Geometry check sheet. Reference: the model listing, model coordinates, mm. A direction names the side the tool comes from. Give positions to 0.01 mm unless a question says otherwise; leave off trailing zeros. Loops run counter-clockwise (first coordinate to the right, second up) from the corner with the lowest first, then second, coordinate; pieces in that order, holes last. Notation, with made-up numbers: (-18.5, 61.25) - (-2.5, 61.25) arc R20 cw to (-2.5, 73.25) - close; hole circle Ø3 at (33, 87). An arc over 180 degrees is marked (long way). Write item = value, one per line. Start each with the question number.
from build123d import *

# Parameters (mm, degrees)
SKETCH11_R          = 1.75
SKETCH8_R           = 1.75
BOSS_EXTRUDE1_DEPTH = 3.5
FILLET1_R           = 2
FILLET2_R           = 2


with BuildPart() as part:
    # Sweep1: sweep along a path in Sketch1
    with BuildLine(Plane(origin=(0, 0, 0), x_dir=(1, 0, 0), z_dir=(0, 1, 0))) as sweep1_path:
        Line((0, 0), (-4.736065928, -1.093406974))
        ThreePointArc((-4.736065928, -1.093406974), (-5.853544334, -1.285424883), (-6.985576472, -1.349706326))
        Line((-6.985576472, -1.349706326), (-210.672794298, -1.349706326))
        ThreePointArc((-210.672794298, -1.349706326), (-212.323270357, -1.212562341), (-213.928475842, -0.804892082))
        Line((-213.928475842, -0.804892082), (-226.582134244, 3.552111915))
        ThreePointArc((-226.582134244, 3.552111915), (-228.446084779, 3.999606846), (-230.361175351, 4.083221506))
        Line((-230.361175351, 4.083221506), (-249.305198661, 3.090407314))
        ThreePointArc((-249.305198661, 3.090407314), (-251.788897094, 2.641281474), (-254.081031741, 1.584592928))
        Line((-254.081031741, 1.584592928), (-268.848792164, -7.643327957))
    # Sketch11 → Sweep1 (sweep)
    with BuildSketch(Plane(origin=(0, 0, 0), x_dir=(0.22495105434386561, 0, 0.9743700647852351), z_dir=(-0.9743700647852351, 0, 0.22495105434386561))):
        Circle(SKETCH11_R)
    sweep(path=sweep1_path.line)

    # Sweep3: sweep along a curve in space
    with BuildLine() as sweep3_path:
        Line((-272.410594168, -3, 9.868988866), (-272.410594168, -8, 9.868988866))
        ThreePointArc((-269.866449879, 0, 8.279231074), (-271.665431558, -0.878679656, 9.403359589), (-272.410594168, -3, 9.868988866))
        Line((-269.866449879, 0, 8.279231074), (-268.848792164, 0, 7.643327957))
    # Sketch8 → Sweep3 (sweep)
    with BuildSketch(Plane(origin=(-196.787061579, 0, 122.966203633), x_dir=(0.5299192642332071, 0, 0.8480480961564246), z_dir=(-0.8480480961564246, 0, 0.5299192642332071))):
        with Locations((-135.986244411, 0)):
            Circle(SKETCH8_R)
    sweep(path=sweep3_path.line)

    # Sketch5 → Boss-Extrude1 (add, symmetric)
    with BuildSketch(Plane(origin=(0, 0, 0), x_dir=(1, 0, 0), z_dir=(0, 1, 0))):
        with BuildLine():
            Line((-0.393664345, 1.705147613), (19.813870271, 14.370895509))
            ThreePointArc((19.813870271, 14.370895509), (20.700469104, 14.828681695), (21.650674926, 15.133205221))
            Line((21.650674926, 15.133205221), (62.574217647, 24.581149504))
            ThreePointArc((62.574217647, 24.581149504), (64.838828602, 24.202183598), (66.172181004, 22.332892472))
            Line((66.172181004, 22.332892472), (69.265258001, 8.935304082))
            ThreePointArc((69.265258001, 8.935304082), (68.886292095, 6.670693126), (67.01700097, 5.337340724))
            Line((67.01700097, 5.337340724), (26.093458249, -4.110603558))
            ThreePointArc((26.093458249, -4.110603558), (25.105924586, -4.253442442), (24.108374578, -4.230646291))
            Line((24.108374578, -4.230646291), (0.393664345, -1.705147613))
            Line((0.393664345, -1.705147613), (-0.393664345, 1.705147613))
        make_face()
    extrude(amount=BOSS_EXTRUDE1_DEPTH, both=True)

    # Fillet1
    # the kernel refuses this fillet: 2 mm, written as the material it takes off along each edge
    with BuildSketch(Plane(origin=(23.000381252, 3.5, -9.286984832), x_dir=(-0.5310851635150788, 0, -0.8473184460957769), z_dir=(-0.8473184460957769, 0, 0.5310851635150788))) as fillet1_piece_1:
        with BuildLine():
            CenterArc((6 - FILLET1_R, FILLET1_R), FILLET1_R, 270, 90)
            Line((6, FILLET1_R), (6, 0))
            Line((6, 0), (6 - FILLET1_R, 0))
        make_face()
    revolve(axis=Axis((23.000381252, 3.5, -9.286984832), (0, -1, 0)), revolution_arc=19.078804313, mode=Mode.SUBTRACT)
    with BuildSketch(Plane(origin=(-4.630256576, 3.5, 0.950278204), x_dir=(0, -1, 0), z_dir=(0.8473184460957748, 0, -0.5310851635150823))) as fillet1_piece_2_section:
        with BuildLine():
            CenterArc((FILLET1_R, -FILLET1_R), FILLET1_R, 90, 90)
            Line((0, -FILLET1_R), (0, 0))
            Line((0, 0), (FILLET1_R, 0))
        make_face()
    fillet1_piece_2 = extrude(amount=28.848807622, mode=Mode.PRIVATE)
    fillet1_piece_2 = split(fillet1_piece_2, bisect_by=Plane(origin=(-1.099290547, 3.044511154, -4.761550481), z_dir=(0.9743700647852351, 0, -0.22495105434386561)), keep=Keep.TOP, mode=Mode.PRIVATE)
    add(fillet1_piece_2, mode=Mode.SUBTRACT)
    with BuildSketch(Plane(origin=(1.518419617, 3.5, 6.576997937), x_dir=(0, -1, 0), z_dir=(-0.22495105434386561, 0, -0.9743700647852351))) as fillet1_piece_3_section:
        with BuildLine():
            CenterArc((FILLET1_R, -FILLET1_R), FILLET1_R, 90, 90)
            Line((0, -FILLET1_R), (0, 0))
            Line((0, 0), (FILLET1_R, 0))
        make_face()
    fillet1_piece_3 = extrude(amount=13.5, mode=Mode.PRIVATE)
    fillet1_piece_3 = fillet1_piece_3 - Plane(origin=(0.460325238, 0, -0.106274455), x_dir=(0.22495105434386553, 0, 0.9743700647852351), z_dir=(-0.9743700647852351, 0, 0.22495105434386553)) * Cylinder(1.75, 36, mode=Mode.PRIVATE)
    add(fillet1_piece_3, mode=Mode.SUBTRACT)
    with BuildSketch(Plane(origin=(24.108374578, 3.5, 4.230646291), x_dir=(0, -1, 0), z_dir=(-0.9943771868431155, 0, -0.10589622413463053))) as fillet1_piece_4_section:
        with BuildLine():
            CenterArc((FILLET1_R, -FILLET1_R), FILLET1_R, 90, 90)
            Line((0, -FILLET1_R), (0, 0))
            Line((0, 0), (FILLET1_R, 0))
        make_face()
    fillet1_piece_4 = extrude(amount=28.848807622, mode=Mode.PRIVATE)
    fillet1_piece_4 = split(fillet1_piece_4, bisect_by=Plane(origin=(1.099289941, 3.044511564, 4.761547859), z_dir=(0.9743700647852351, 0, -0.22495105434386561)), keep=Keep.TOP, mode=Mode.PRIVATE)
    add(fillet1_piece_4, mode=Mode.SUBTRACT)
    with BuildSketch(Plane(origin=(24.743751923, 3.5, -1.73561683), x_dir=(0.22495105434386634, 0, 0.9743700647852349), z_dir=(0.9743700647852349, 0, -0.22495105434386634))) as fillet1_piece_5:
        with BuildLine():
            CenterArc((6 - FILLET1_R, FILLET1_R), FILLET1_R, 270, 90)
            Line((6, FILLET1_R), (6, 0))
            Line((6, 0), (6 - FILLET1_R, 0))
        make_face()
    revolve(axis=Axis((24.743751923, 3.5, -1.73561683), (0, -1, 0)), revolution_arc=19.078804313, mode=Mode.SUBTRACT)
    with BuildSketch(Plane(origin=(67.01700097, 3.5, -5.337340724), x_dir=(-0.22495105434386584, 0, -0.9743700647852351), z_dir=(-0.9743700647852351, 0, 0.22495105434386584)), Plane(origin=(21.650674926, 3.5, -15.133205221), x_dir=(0.22495105434386575, 0, 0.974370064785235), z_dir=(0.9743700647852351, 0, -0.22495105434386578))) as fillet1_piece_6:
        with BuildLine():
            CenterArc((FILLET1_R, FILLET1_R), FILLET1_R, 180, 90)
            Line((0, FILLET1_R), (0, 0))
            Line((0, 0), (FILLET1_R, 0))
        make_face()
    extrude(amount=42, mode=Mode.SUBTRACT)
    with BuildSketch(Plane(origin=(66.342147807, 3.5, -8.260450918), x_dir=(0.9743700647852359, 0, -0.22495105434386237), z_dir=(-0.22495105434386237, 0, -0.9743700647852359))) as fillet1_piece_7:
        with BuildLine():
            CenterArc((3 - FILLET1_R, FILLET1_R), FILLET1_R, 270, 90)
            Line((3, FILLET1_R), (3, 0))
            Line((3, 0), (3 - FILLET1_R, 0))
        make_face()
    revolve(axis=Axis((66.342147807, 3.5, -8.260450918), (0, -1, 0)), revolution_arc=90, mode=Mode.SUBTRACT)
    with BuildSketch(Plane(origin=(66.172181004, 3.5, -22.332892472), x_dir=(-0.9743700647852351, 0, 0.22495105434386561), z_dir=(0.2249510543438656, 0, 0.9743700647852351))) as fillet1_piece_8:
        with BuildLine():
            CenterArc((FILLET1_R, FILLET1_R), FILLET1_R, 180, 90)
            Line((0, FILLET1_R), (0, 0))
            Line((0, 0), (FILLET1_R, 0))
        make_face()
    extrude(amount=13.75, mode=Mode.SUBTRACT)
    with BuildSketch(Plane(origin=(63.24907081, 3.5, -21.658039309), x_dir=(-0.22495105434387033, 0, -0.974370064785234), z_dir=(-0.974370064785234, 0, 0.22495105434387033))) as fillet1_piece_9:
        with BuildLine():
            CenterArc((3 - FILLET1_R, FILLET1_R), FILLET1_R, 270, 90)
            Line((3, FILLET1_R), (3, 0))
            Line((3, 0), (3 - FILLET1_R, 0))
        make_face()
    revolve(axis=Axis((63.24907081, 3.5, -21.658039309), (0, -1, 0)), revolution_arc=90, mode=Mode.SUBTRACT)

    # Fillet2
    # the kernel refuses this fillet: 2 mm, written as the material it takes off along each edge
    with BuildSketch(Plane(origin=(23.000381252, -3.5, -9.286984832), x_dir=(-0.5310851635150788, 0, -0.8473184460957769), z_dir=(-0.8473184460957769, 0, 0.5310851635150788))) as fillet2_piece_1:
        with BuildLine():
            CenterArc((6 - FILLET2_R, -FILLET2_R), FILLET2_R, 0, 90)
            Line((6, -FILLET2_R), (6, 0))
            Line((6, 0), (6 - FILLET2_R, 0))
        make_face()
    revolve(axis=Axis((23.000381252, -3.5, -9.286984832), (0, -1, 0)), revolution_arc=19.078804313, mode=Mode.SUBTRACT)
    with BuildSketch(Plane(origin=(-4.630256576, -3.5, 0.950278204), x_dir=(0, 1, 0), z_dir=(0.8473184460957748, 0, -0.5310851635150823))) as fillet2_piece_2_section:
        with BuildLine():
            CenterArc((FILLET2_R, FILLET2_R), FILLET2_R, 180, 90)
            Line((0, FILLET2_R), (0, 0))
            Line((0, 0), (FILLET2_R, 0))
        make_face()
    fillet2_piece_2 = extrude(amount=28.848807622, mode=Mode.PRIVATE)
    fillet2_piece_2 = split(fillet2_piece_2, bisect_by=Plane(origin=(-1.099290547, -3.044511154, -4.761550481), z_dir=(0.9743700647852351, 0, -0.22495105434386561)), keep=Keep.TOP, mode=Mode.PRIVATE)
    add(fillet2_piece_2, mode=Mode.SUBTRACT)
    with BuildSketch(Plane(origin=(1.518419617, -3.5, 6.576997937), x_dir=(0, 1, 0), z_dir=(-0.22495105434386561, 0, -0.9743700647852351))) as fillet2_piece_3_section:
        with BuildLine():
            CenterArc((FILLET2_R, FILLET2_R), FILLET2_R, 180, 90)
            Line((0, FILLET2_R), (0, 0))
            Line((0, 0), (FILLET2_R, 0))
        make_face()
    fillet2_piece_3 = extrude(amount=13.5, mode=Mode.PRIVATE)
    fillet2_piece_3 = fillet2_piece_3 - Plane(origin=(0.460325238, 0, -0.106274455), x_dir=(0.22495105434386553, 0, 0.9743700647852351), z_dir=(-0.9743700647852351, 0, 0.22495105434386553)) * Cylinder(1.75, 36, mode=Mode.PRIVATE)
    add(fillet2_piece_3, mode=Mode.SUBTRACT)
    with BuildSketch(Plane(origin=(24.108374578, -3.5, 4.230646291), x_dir=(0, 1, 0), z_dir=(-0.9943771868431155, 0, -0.10589622413463053))) as fillet2_piece_4_section:
        with BuildLine():
            CenterArc((FILLET2_R, FILLET2_R), FILLET2_R, 180, 90)
            Line((0, FILLET2_R), (0, 0))
            Line((0, 0), (FILLET2_R, 0))
        make_face()
    fillet2_piece_4 = extrude(amount=28.848807622, mode=Mode.PRIVATE)
    fillet2_piece_4 = split(fillet2_piece_4, bisect_by=Plane(origin=(1.099289941, -3.044511564, 4.761547859), z_dir=(0.9743700647852351, 0, -0.22495105434386561)), keep=Keep.TOP, mode=Mode.PRIVATE)
    add(fillet2_piece_4, mode=Mode.SUBTRACT)
    with BuildSketch(Plane(origin=(24.743751923, -3.5, -1.73561683), x_dir=(0.22495105434386634, 0, 0.9743700647852349), z_dir=(0.9743700647852349, 0, -0.22495105434386634))) as fillet2_piece_5:
        with BuildLine():
            CenterArc((6 - FILLET2_R, -FILLET2_R), FILLET2_R, 0, 90)
            Line((6, -FILLET2_R), (6, 0))
            Line((6, 0), (6 - FILLET2_R, 0))
        make_face()
    revolve(axis=Axis((24.743751923, -3.5, -1.73561683), (0, -1, 0)), revolution_arc=19.078804313, mode=Mode.SUBTRACT)
    with BuildSketch(Plane(origin=(67.01700097, -3.5, -5.337340724), x_dir=(-0.22495105434386584, 0, -0.9743700647852351), z_dir=(-0.9743700647852351, 0, 0.22495105434386584)), Plane(origin=(21.650674926, -3.5, -15.133205221), x_dir=(0.22495105434386575, 0, 0.974370064785235), z_dir=(0.9743700647852351, 0, -0.22495105434386578))) as fillet2_piece_6:
        with BuildLine():
            CenterArc((FILLET2_R, -FILLET2_R), FILLET2_R, 90, 90)
            Line((0, -FILLET2_R), (0, 0))
            Line((0, 0), (FILLET2_R, 0))
        make_face()
    extrude(amount=42, mode=Mode.SUBTRACT)
    with BuildSketch(Plane(origin=(66.342147807, -3.5, -8.260450918), x_dir=(0.9743700647852359, 0, -0.22495105434386237), z_dir=(-0.22495105434386237, 0, -0.9743700647852359))) as fillet2_piece_7:
        with BuildLine():
            CenterArc((3 - FILLET2_R, -FILLET2_R), FILLET2_R, 0, 90)
            Line((3, -FILLET2_R), (3, 0))
            Line((3, 0), (3 - FILLET2_R, 0))
        make_face()
    revolve(axis=Axis((66.342147807, -3.5, -8.260450918), (0, -1, 0)), revolution_arc=90, mode=Mode.SUBTRACT)
    with BuildSketch(Plane(origin=(66.172181004, -3.5, -22.332892472), x_dir=(-0.9743700647852351, 0, 0.22495105434386561), z_dir=(0.2249510543438656, 0, 0.9743700647852351))) as fillet2_piece_8:
        with BuildLine():
            CenterArc((FILLET2_R, -FILLET2_R), FILLET2_R, 90, 90)
            Line((0, -FILLET2_R), (0, 0))
            Line((0, 0), (FILLET2_R, 0))
        make_face()
    extrude(amount=13.75, mode=Mode.SUBTRACT)
    with BuildSketch(Plane(origin=(63.24907081, -3.5, -21.658039309), x_dir=(-0.22495105434387033, 0, -0.974370064785234), z_dir=(-0.974370064785234, 0, 0.22495105434387033))) as fillet2_piece_9:
        with BuildLine():
            CenterArc((3 - FILLET2_R, -FILLET2_R), FILLET2_R, 0, 90)
            Line((3, -FILLET2_R), (3, 0))
            Line((3, 0), (3 - FILLET2_R, 0))
        make_face()
    revolve(axis=Axis((63.24907081, -3.5, -21.658039309), (0, -1, 0)), revolution_arc=90, mode=Mode.SUBTRACT)


solid = part.part
1) Gauge pin test, flat ends, axial feed: P1, Ø5, axis at x = -157.5, y = 1.5, coming from the +Z side; P2, Ø2, axis at x = -189.5, y = -0.5, coming from the -Z side; P3, Ø20, axis at x = 49, z = -11, coming from the -Y side; P4, Ø1, axis at x = -57, z = -2.5, coming from the -Y side. Record the tip position at first contact, or that the pin passes through.
2) Material ranges on line 1 along Y through (x, z) = (45.5, -15); line 2 along Z through (x, y) = (-35, -1.5); line 3 along Z through (x, y) = (0, -1.5), recorded low to high.
3) Tool access check on faces 4 (the face through (42, 3.5, -10)), 5 (the face through (9.57, 0.02, -7.95)). Record the directions out of +Z, -Z, +X, -X, +Y, -Y that give a thin tool (end or side, any length) a straight path to the whole face; none if there is none.
4) Cross-section at A-A on x = -135. Enter the section's corners in (y, z).
5) Release check for a two-part mould opening along X. For faces 1 (the face through (41.83, 0.02, -19.79)), 2 (the face through (-220.89, 0.53, 0.17)), 3 (the face through (46.84, 0.02, -0.68)) record: pulls with the +X half, pulls with the -X half, needs draft (parallel to the pull), parting line crosses it, or undercut.
Checked values:
q1.P1 = 3.1
q1.P2 = -0.4
q1.P3 = -3.5
q1.P4 = through
q2.line_1 = -3.5 to 3.5
q2.line_2 = 0.45 to 2.25
q2.line_3 = -1.95 to 0.93
q3.face_4 = +Z, -Z, +X, -X, +Y
q3.face_5 = -Z, +Y, -Y
q4.outline = circle Ø3.5 at (0, 1.35)
q5.face_1 = pulls with the -X half
q5.face_2 = undercut
q5.face_3 = pulls with the +X half
